Geometry: final body of the model. Coordinates: model frame, mm. Give positions to 0.01 mm unless a question says otherwise; leave off trailing zeros. Loops run counter-clockwise (first coordinate to the right, second up) from the corner with the lowest first, then second, coordinate; pieces in that order, holes last.
```python
from build123d import *

# Parameters (mm, degrees)
F0_W         = 6
F0_H         = 35
F0_R         = 1.65
F0_R_2       = 1
F1_DEPTH     = 1.5
F2_R         = 2
F3_T1_DEPTH  = 31
F3_T3_DEPTH  = 2
F3_T6_ANGLE  = 90
F3_T8_ANGLE  = 90
F3_T10_ANGLE = 90
F3_T12_ANGLE = 90
F3_T14_ANGLE = 90
F3_T16_ANGLE = 90
F3_T18_ANGLE = 90
F3_T20_ANGLE = 90


# Not quite as in the source:
# - a fillet or chamfer that OpenCascade refuses, or shapes differently, is made with other operations: its cross-section is extruded or revolved along the edge and cut away or added


with BuildPart() as f1:
    # F0 (on Top) → F1 (new body)
    with BuildSketch(Plane.XY):
        Rectangle(F0_W, F0_H)
        with Locations((0.0021975506, -14.9999999195)):
            Circle(F0_R, mode=Mode.SUBTRACT)
        with Locations((0.0021975506, -9)):
            Circle(F0_R_2, mode=Mode.SUBTRACT)
        with Locations((0, 9)):
            Circle(F0_R_2, mode=Mode.SUBTRACT)
        with Locations((0, 15)):
            Circle(F0_R, mode=Mode.SUBTRACT)
    extrude(amount=F1_DEPTH)

    # F2
    f2_edges = [f1.edges().sort_by_distance(p)[0] for p in [
        (-3, 17.5, 0.75),
        (3, 17.5, 0.75),
        (-3, -17.5, 0.75),
        (3, -17.5, 0.75),
    ]]
    fillet(f2_edges, radius=F2_R)

    # F3: chamfer of 0.5 on 22 edges, made by hand

    # F3_s2 → F3_t1 (cut)
    with BuildSketch(Plane.XZ.offset(-15.5)):
        Polygon((-2.5, 1.5), (-3, 1), (-3, 1.5), align=None)
        Polygon((2.5, 1.5), (3, 1), (3, 1.5), align=None)
        Polygon((2.5, 0), (3, 0.5), (3, 0), align=None)
        Polygon((-2.5, 0), (-3, 0.5), (-3, 0), align=None)
    extrude(amount=F3_T1_DEPTH, mode=Mode.SUBTRACT)

    # F3_s4 → F3_t3 (cut)
    with BuildSketch(Plane.YZ.offset(-1)):
        Polygon((17.5, 1), (17, 1.5), (17.5, 1.5), align=None)
        Polygon((-17, 1.5), (-17.5, 1), (-17.5, 1.5), align=None)
        Polygon((17.5, 0.5), (17, 0), (17.5, 0), align=None)
        Polygon((-17, 0), (-17.5, 0.5), (-17.5, 0), align=None)
    extrude(amount=F3_T3_DEPTH, mode=Mode.SUBTRACT)

    # F3_s5 → F3_t6 (revolve, cut)
    with BuildSketch(Plane.YZ.offset(1)):
        Polygon((17.5, 1), (17, 1.5), (17.5, 1.5), align=None)
    revolve(axis=Axis((1, 15.5, 1.5), (0, 0, -1)), revolution_arc=F3_T6_ANGLE, mode=Mode.SUBTRACT)

    # F3_s7 → F3_t8 (revolve, cut)
    with BuildSketch(Plane.YZ.offset(-1)):
        Polygon((17.5, 1), (17, 1.5), (17.5, 1.5), align=None)
    revolve(axis=Axis((-1, 15.5, 1.5), (0, 0, 1)), revolution_arc=F3_T8_ANGLE, mode=Mode.SUBTRACT)

    # F3_s9 → F3_t10 (revolve, cut)
    with BuildSketch(Plane.XZ.offset(15.5)):
        Polygon((-2.5, 1.5), (-3, 1), (-3, 1.5), align=None)
    revolve(axis=Axis((-1, -15.5, 1.5), (0, 0, 1)), revolution_arc=F3_T10_ANGLE, mode=Mode.SUBTRACT)

    # F3_s11 → F3_t12 (revolve, cut)
    with BuildSketch(Plane.YZ.offset(1)):
        Polygon((-17, 1.5), (-17.5, 1), (-17.5, 1.5), align=None)
    revolve(axis=Axis((1, -15.5, 1.5), (0, 0, 1)), revolution_arc=F3_T12_ANGLE, mode=Mode.SUBTRACT)

    # F3_s13 → F3_t14 (revolve, cut)
    with BuildSketch(Plane.YZ.offset(-1)):
        Polygon((17, 0), (17.5, 0.5), (17.5, 0), align=None)
    revolve(axis=Axis((-1, 15.5, 0), (0, 0, 1)), revolution_arc=F3_T14_ANGLE, mode=Mode.SUBTRACT)

    # F3_s15 → F3_t16 (revolve, cut)
    with BuildSketch(Plane.YZ.offset(1)):
        Polygon((17, 0), (17.5, 0.5), (17.5, 0), align=None)
    revolve(axis=Axis((1, 15.5, 0), (0, 0, -1)), revolution_arc=F3_T16_ANGLE, mode=Mode.SUBTRACT)

    # F3_s17 → F3_t18 (revolve, cut)
    with BuildSketch(Plane.XZ.offset(15.5)):
        Polygon((-2.5, 0), (-3, 0.5), (-3, 0), align=None)
    revolve(axis=Axis((-1, -15.5, 0), (0, 0, 1)), revolution_arc=F3_T18_ANGLE, mode=Mode.SUBTRACT)

    # F3_s19 → F3_t20 (revolve, cut)
    with BuildSketch(Plane.YZ.offset(1)):
        Polygon((-17, 0), (-17.5, 0.5), (-17.5, 0), align=None)
    revolve(axis=Axis((1, -15.5, 0), (0, 0, 1)), revolution_arc=F3_T20_ANGLE, mode=Mode.SUBTRACT)

    # F3_s21 → F3_t22 (revolve, cut)
    with BuildSketch(Plane.XZ.offset(9)):
        Polygon((1.5021975506, 0), (1.0021975506, 0.5), (1.0021975506, 0), align=None)
    revolve(axis=Axis((0.0021975506, -9, 0), (0, 0, 1)), mode=Mode.SUBTRACT)

    # F3_s23 → F3_t24 (revolve, cut)
    with BuildSketch(Plane.XZ.offset(-9)):
        Polygon((1.5, 0), (1, 0.5), (1, 0), align=None)
    revolve(axis=Axis((0, 9, 0), (0, 0, 1)), mode=Mode.SUBTRACT)

    # F3_s25 → F3_t26 (revolve, cut)
    with BuildSketch(Plane.XZ.offset(-15)):
        Polygon((2.15, 0), (1.65, 0.5), (1.65, 0), align=None)
    revolve(axis=Axis((0, 15, 0), (0, 0, 1)), mode=Mode.SUBTRACT)

    # F3_s27 → F3_t28 (revolve, cut)
    with BuildSketch(Plane.XZ.offset(9)):
        Polygon((1.5021975506, 1.5), (1.0021975506, 1), (1.0021975506, 1.5), align=None)
    revolve(axis=Axis((0.0021975506, -9, 1.5), (0, 0, 1)), mode=Mode.SUBTRACT)

    # F3_s29 → F3_t30 (revolve, cut)
    with BuildSketch(Plane.XZ.offset(14.9999999195)):
        Polygon((2.1521975506, 1.5), (1.6521975506, 1), (1.6521975506, 1.5), align=None)
    revolve(axis=Axis((0.0021975506, -14.9999999195, 1.5), (0, 0, 1)), mode=Mode.SUBTRACT)

    # F3_s31 → F3_t32 (revolve, cut)
    with BuildSketch(Plane.XZ.offset(14.9999999195)):
        Polygon((2.1521975506, 0), (1.6521975506, 0.5), (1.6521975506, 0), align=None)
    revolve(axis=Axis((0.0021975506, -14.9999999195, 0), (0, 0, 1)), mode=Mode.SUBTRACT)


solid = f1.part
```
Q1. Mould query, pull axis X, two halves, no side actions, for faces 1 (the face through (-2.17, -16.65, 1.36)), 2 (the face through (0, 0, 0)), 3 (the face through (2.15, -16.67, 0.14)), 4 (the face through (-0.13, -8.01, 0.75)). Classes: +X half, -X half, draft (parallel to the pull), parting line (faces both ways), or undercut.
Q2. Section query A-A, the plane y = 15. Return loops of the section in (x, z), and give its area (3 significant figures).
Q3. Material intervals for probe 1 along Y at (x, z) = (-1.5, 0.95); probe 2 along Y at (x, z) = (0, 1.2); probe 3 along Y at (x, z) = (1.25, 0.7), sorted ascending.
Q4. Section query B-B, the plane z = 0.75. Return loops of the section in (x, y), and give its area (3 significant figures).
Q5. Section query C-C, the plane y = 9. Return loops of the section in (x, z).
Q6. Section query D-D, the plane x = 0. State how many separate pieces and enclosed holes the cut face has, and give its area (3 significant figures).
Resolved:
1. face 1: -X half
1. face 2: draft
1. face 3: +X half
1. face 4: undercut
2. outline: (-3, 0.5) - (-2.5, 0) - (-2.15, 0) - (-1.65, 0.5) - (-1.65, 1.5) - (-2.5, 1.5) - (-3, 1) - close; (1.65, 0.5) - (2.15, 0) - (2.5, 0) - (3, 0.5) - (3, 1) - (2.5, 1.5) - (1.65, 1.5) - close
2. area: 3.30 mm2
3. probe 1: y = -17.44 to -15.68, -14.32 to 14.31, 15.69 to 17.44
3. probe 2: y = -17.3 to -16.85, -13.15 to -10.2, -7.8 to 8, 10 to 13.35, 16.65 to 17.3
3. probe 3: y = -17.48 to -16.08, -13.92 to 13.92, 16.08 to 17.48
4. outline: (-3, -15.5) arc R2 ccw to (-1, -17.5) - (1, -17.5) arc R2 ccw to (3, -15.5) - (3, 15.5) arc R2 ccw to (1, 17.5) - (-1, 17.5) arc R2 ccw to (-3, 15.5) - close; hole circle Ø3.3 at (0, -15); hole circle Ø3.3 at (0, 15); hole circle Ø2 at (0, -9); hole circle Ø2 at (0, 9)
4. area: 183 mm2
5. outline: (-3, 0.5) - (-2.5, 0) - (-1.5, 0) - (-1, 0.5) - (-1, 1.5) - (-2.5, 1.5) - (-3, 1) - close; (1, 0.5) - (1.5, 0) - (2.5, 0) - (3, 0.5) - (3, 1) - (2.5, 1.5) - (1, 1.5) - close
6. separate pieces: 5
6. enclosed holes: 0
6. area: 34.6 mm2
